Work out the finished part from the listing and answer in its coordinate system (mm). Face numbers are marked on the shaded views. Coordinates: 2 decimals unless noted, no trailing zeros. Write each loop counter-clockwise with the first axis right and the second up, starting at its lowest first coordinate (ties: lowest second). Pieces come first, ordered by that corner, then holes. Notation, with made-up numbers: (-1.75, 13) -> (35.25, 13) arc R16 ccw to (35.25, 38) -> close; hole circle Ø11 at (24, 37). An arc over 180 degrees is marked (long way). Write each question's results on one line, items separated by ' | '. Start each with the question number.
from build123d import *

# Parameters (mm, degrees)
SKETCH1_W                                       = 38.677516632
SKETCH1_H                                       = 80.9364214
BOSS_EXTRUDE1_DEPTH                             = 5
FILLET1_R                                       = 10
BOSS_EXTRUDE2_DEPTH                             = 19.8
CHAMFER1_SIZE                                   = 1
CSK_FOR_M2_FLAT_HEAD_MACHINE_SCREW1_D           = 2.4
CSK_FOR_M2_FLAT_HEAD_MACHINE_SCREW1_CSINK_D     = 4.4
CSK_FOR_M2_FLAT_HEAD_MACHINE_SCREW1_CSINK_ANGLE = 90
CUT_EXTRUDE3_REACH                              = 63.226
SKETCH12_W                                      = 9.354156198
SKETCH12_H                                      = 8.387423898
CHAMFER3_SIZE                                   = 1
SKETCH15_R                                      = 1.2
CUT_EXTRUDE4_DEPTH                              = 10


with BuildPart() as part:
    # Sketch1 → Boss-Extrude1 (new body)
    # profile 1 of 2: a face of its own
    with BuildSketch(Plane(origin=(0, 0, 0), x_dir=(1, 0, 0), z_dir=(0, 1, 0))):
        with Locations((19.338758316, 0)):
            Rectangle(SKETCH1_W, SKETCH1_H)
        Polygon((25.6, 34.765367903), (27.2, 31.994086611), (25.6, 29.222805318), (22.4, 29.222805318), (20.8, 31.994086611), (22.4, 34.765367903), align=None, mode=Mode.SUBTRACT)
    # profile 2 of 2: a face of its own
    with BuildSketch(Plane(origin=(0, 0, 0), x_dir=(1, 0, 0), z_dir=(0, 1, 0))):
        with Locations((-19.338758316, 0)):
            Rectangle(SKETCH1_W, SKETCH1_H)
        Polygon((-24, 35.251299163), (-21.228718708, 33.651299163), (-21.228718708, 30.451299163), (-24, 28.851299163), (-26.771281292, 30.451299163), (-26.771281292, 33.651299163), align=None, mode=Mode.SUBTRACT)
    extrude(amount=BOSS_EXTRUDE1_DEPTH)

    # Fillet1
    fillet1_edges = [part.edges().sort_by_distance(p)[0] for p in [
        (-38.677516632, 2.5, 40.4682107),
        (-38.677516632, 2.5, -40.4682107),
        (38.677516632, 2.5, -40.4682107),
        (38.677516632, 2.5, 40.4682107),
    ]]
    fillet(fillet1_edges, radius=FILLET1_R)

    # Sketch7 → Boss-Extrude2 (add)
    # profile 1 of 2: a face of its own
    with BuildSketch(Plane(origin=(0, 5, 0), x_dir=(1, 0, 0), z_dir=(0, 1, 0))):
        Polygon((-18.728718708, 35.094674836), (-24, 38.138050509), (-29.271281292, 35.094674836), (-29.271281292, 29.00792349), (-24, 25.964547817), (-18.728718708, 29.00792349), align=None)
        Polygon((-21.228718708, 30.451299163), (-21.228718708, 33.651299163), (-24, 35.251299163), (-26.771281292, 33.651299163), (-26.771281292, 30.451299163), (-24, 28.851299163), align=None, mode=Mode.SUBTRACT)
    # profile 2 of 2: a face of its own
    with BuildSketch(Plane(origin=(0, 5, 0), x_dir=(1, 0, 0), z_dir=(0, 1, 0))):
        Polygon((27.043375673, 37.265367903), (20.956624327, 37.265367903), (17.913248654, 31.994086611), (20.956624327, 26.722805318), (27.043375673, 26.722805318), (30.086751346, 31.994086611), align=None)
        Polygon((25.6, 34.765367903), (22.4, 34.765367903), (20.8, 31.994086611), (22.4, 29.222805318), (25.6, 29.222805318), (27.2, 31.994086611), align=None, mode=Mode.SUBTRACT)
    extrude(amount=BOSS_EXTRUDE2_DEPTH)

    # Chamfer1
    chamfer1_edges = [part.edges().sort_by_distance(p)[0] for p in [
        (-18.728718708, 5, -32.051299163),
        (-21.364359354, 5, -36.616362672),
        (-26.635640646, 5, -36.616362672),
        (-29.271281292, 5, -32.051299163),
        (-26.635640646, 5, -27.486235653),
        (-21.364359354, 5, -27.486235653),
        (28.565063509, 5, -34.629727257),
        (24, 5, -37.265367903),
        (19.434936491, 5, -34.629727257),
        (19.434936491, 5, -29.358445964),
        (24, 5, -26.722805318),
        (28.565063509, 5, -29.358445964),
    ]]
    chamfer(chamfer1_edges, length=CHAMFER1_SIZE)

    # CSK for M2 Flat Head Machine Screw1 (through all)
    with Locations(Plane(origin=(0, 0, 0), x_dir=(-1, 0, 0), z_dir=(0, -1, 0))):
        with Locations((-25, -5.898372583), (0, -30.898372583), (23.5, -5.898372583), (0, 19.101627417)):
            CounterSinkHole(CSK_FOR_M2_FLAT_HEAD_MACHINE_SCREW1_D / 2, CSK_FOR_M2_FLAT_HEAD_MACHINE_SCREW1_CSINK_D / 2, counter_sink_angle=CSK_FOR_M2_FLAT_HEAD_MACHINE_SCREW1_CSINK_ANGLE)

    # Sketch12 → Cut-Extrude3 (cut, up to next)
    with BuildSketch(Plane.XZ, mode=Mode.PRIVATE) as cut_extrude3_sk1:
        with Locations((4.598685832, 16.15981243)):
            Rectangle(SKETCH12_W, SKETCH12_H)
    cut_extrude3_tool1 = extrude(cut_extrude3_sk1.sketch, amount=-CUT_EXTRUDE3_REACH, mode=Mode.PRIVATE) & part.part
    add(cut_extrude3_tool1.solids().sort_by_distance((4.598686, 0, 16.159812))[0], mode=Mode.SUBTRACT)

    # Chamfer3
    chamfer3_edges = [part.edges().sort_by_distance(p)[0] for p in [
        (9.275763931, 2.5, 20.353524379),
        (9.275763931, 2.5, 11.966100481),
        (-0.078392267, 2.5, 11.966100481),
        (-0.078392267, 2.5, 20.353524379),
    ]]
    chamfer(chamfer3_edges, length=CHAMFER3_SIZE)

    # Sketch15 → Cut-Extrude4 (cut)
    with BuildSketch(Plane(origin=(0, 5, 0), x_dir=(1, 0, 0), z_dir=(0, 1, 0))):
        with Locations(Location((16.71400844, -10.060201476, 0), (0, 0, 270))):
            Circle(SKETCH15_R)
        with Locations(Location((16.71400844, 0.06847889, 0), (0, 0, 270))):
            Circle(SKETCH15_R)
    extrude(amount=-CUT_EXTRUDE4_DEPTH, mode=Mode.SUBTRACT)


solid = part.part
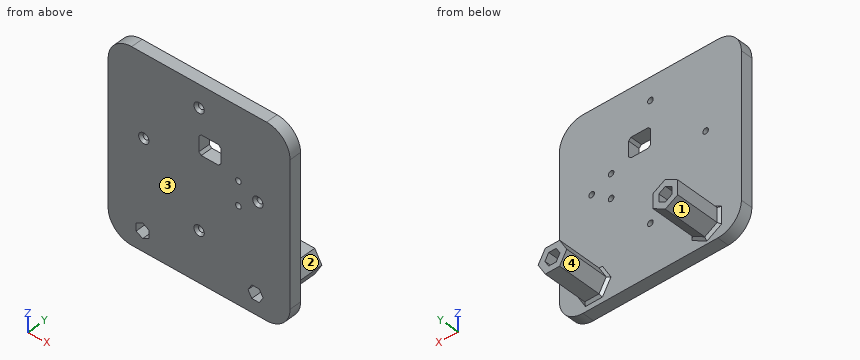
1. Find section C-C on x = -5.5. Give the vertices of the cut face in (y, z).
2. Given pin 1 Ø10 at (x, z) = (-28, 30.5) entering from -Y; pin 2 Ø5 at (x, y) = (-19, 15) entering from +Z; pin 3 Ø4 at (x, y) = (-27, 20.5) entering from +Z; pin 4 Ø5 at (x, y) = (23, 14.5) entering from +Z, each flat-ended and moving along its own axis, determine where each tip first touches the part or whether it passes through.
3. Find section A-A on y = 17. Give the vertices of the cut face in (x, z), and give its area (3 significant figures).
4. Determine the mould class of the marked faces 1, 2, 3 and 4 for opening direction X: pulls with the +X half, pulls with the -X half, needs draft (parallel to the pull), parting line crosses it, or undercut.
5. Find the intervals of material crossed by L1, parallel to X at y = 23, z = -32; L2, parallel to Y at x = 14, z = 37.5; L3, parallel to Z at x = -23.5, y = 3.95, in increasing order.
6. Find section B-B on x = -20. Give the vertices of the cut face in (y, z), and give its area (3 significant figures).
Ans:
1) outline: (0, -40.47) -> (5, -40.47) -> (5, 40.47) -> (0, 40.47) -> close
2) pin 1: stops at y = 0 | pin 2: stops at z = -27.41 | pin 3: stops at z = -26.54 | pin 4: stops at z = -26.72
3) outline: (-29.27, -35.09) -> (-24, -38.14) -> (-18.73, -35.09) -> (-18.73, -29.01) -> (-24, -25.96) -> (-29.27, -29.01) -> close; (17.91, -31.99) -> (20.96, -37.27) -> (27.04, -37.27) -> (30.09, -31.99) -> (27.04, -26.72) -> (20.96, -26.72) -> close; hole (-26.77, -33.65) -> (-24, -35.25) -> (-21.23, -33.65) -> (-21.23, -30.45) -> (-24, -28.85) -> (-26.77, -30.45) -> close; hole (20.8, -31.99) -> (22.4, -34.77) -> (25.6, -34.77) -> (27.2, -31.99) -> (25.6, -29.22) -> (22.4, -29.22) -> close | area: 139 mm²
4) face 1: pulls with the -X half | face 2: pulls with the +X half | face 3: needs draft | face 4: undercut
5) L1: x = -29.27 to -26.77, -21.23 to -18.73, 17.92 to 20.8, 27.2 to 30.08 | L2: y = 0 to 5 | L3: z = -40.47 to -34.96, -29.14 to 4.7, 7.1 to 40.47
6) outline: (0, -40.47) -> (5, -40.47) -> (5, -36.98) -> (6, -35.83) -> (24.8, -35.83) -> (24.8, -28.27) -> (6, -28.27) -> (5, -27.12) -> (5, 40.47) -> (0, 40.47) -> close | area: 555 mm²
